Here's how the part is built. I have some questions about the finished solid (model axes, mm). Round coordinates to 2 decimals unless told otherwise and drop trailing zeros.
```python
from build123d import *

# Parameters (mm, degrees)
PAD_DEPTH       = 2
POCKET_DEPTH    = 5
SKETCH004_R     = 4.32335
POCKET001_DEPTH = 5
PAD001_DEPTH    = 0.2
FILLET_R        = 0.5


with BuildPart() as part:
    # Sketch → Pad (new body)
    with BuildSketch(Plane.XY):
        with BuildLine():
            Line((-0.976296, -0.21644), (-6.834079, 26.206312))
            ThreePointArc((6.834079, 26.206312), (0, 34.721358), (-6.834079, 26.206312))
            Line((6.834079, 26.206312), (0.976296, -0.21644))
            ThreePointArc((-0.976296, -0.21644), (0, -1), (0.976296, -0.21644))
        make_face()
    extrude(amount=PAD_DEPTH)

    # Sketch001 → Pocket (cut)
    with BuildSketch(Plane(origin=(0.976296, -0.21644, 0), x_dir=(0.21644, 0.976296, 0), z_dir=(0.976296, -0.21644, 0))):
        Polygon((-2, 0.3), (10, 3), (-2, 3), align=None)
    extrude(amount=-POCKET_DEPTH, mode=Mode.SUBTRACT)

    # Sketch004 → Pocket001 (cut)
    with BuildSketch(Plane.XY.offset(2)):
        with Locations((0, 27.84)):
            Circle(SKETCH004_R)
    extrude(amount=-POCKET001_DEPTH, mode=Mode.SUBTRACT)

    # Sketch005 → Pad001 (new body)
    with BuildSketch(Plane.XY.offset(2)):
        Polygon((-3.5, 22.121615), (3.5, 22.121615), (3.5, 17.9142), (2.709286, 17.9142), (1.636494, 21.215913), (0.563703, 17.9142), (-2.907924, 17.9142), (-0.099319, 15.873629), (-0.343663, 15.121615), (-3.5, 15.121615), align=None)
    extrude(amount=PAD001_DEPTH)

    # Fillet
    fillet_edges = [part.edges().sort_by_distance(p)[0] for p in [
        (-4.619025, 16.214851, 2),
    ]]
    fillet(fillet_edges, radius=FILLET_R)


solid = part.part
```
1. If we mould it in two halves opening along X, with no side actions, what happens to faces 1 (the cylindrical face through (0.18, 34.72, 0.74)), 2 (the cylindrical face through (4.124, 29.139, 1.014)), 3 (the cylindrical face through (-4.25, 15.21, 1.85))? For each: released by +X, released by -X, zero draft, split by the parting line, or undercut.
Evaluation:
face 1: split by the parting line
face 2: undercut
face 3: released by -X
2. I'm going to push flat-ended pins straight in: P1, Ø8, axis at x = -4.5, y = 7, coming from the +Z side; P2, Ø1, axis at y = 11, z = 1.5, coming from the +X side. Where does each tip first touch, or does it pass through?
Evaluation:
P1: stops at z = 2
P2: stops at x = 3.57
3. I need wall thicknesses on probe 1 along Z at (x, y) = (3, 11); probe 2 along X at (y, z) = (22, 1.5); probe 3 along X at (y, z) = (23, 0.9). Which ranges of each line are inside material? Lowest first, please.
Evaluation:
probe 1: z = 0 to 2
probe 2: x = -5.9 to 5.9
probe 3: x = -6.12 to 6.12
